Can you work these out from the model? Positions are in its coordinate system, mm. A direction names the side the tool comes from. Give positions to 0.01 mm unless a question says otherwise; leave off trailing zeros. Order: outer loops, then holes, each group sorted by start corner. A loop starts at its lowest first (then second) coordinate and runs counter-clockwise, first axis right, second up. Notation, with made-up numbers: (24.5, 62) - (29.5, 62) arc R12 cw to (29.5, 73) - close; hole circle Ø1 at (34.25, 3.25). An arc over 180 degrees is marked (long way). Use one line per item in the form item = value. Start each with the question number.
1) Which directions (+Z, -Z, +X, -X, +Y, -Y) give clear straight access to the entire face, cutting with the end or side of a thin tool? Please do faces 4 (the flat face through (1.2, -1.2, 5.85)), 5 (the flat face through (-1, -1, 6.35)).
2) Suppose I cut it at C-C, the plane z = 2.5. Write out the boundary of the cut face in (x, y), and give its area (3 significant figures).
3) We'd pull the mould along Y, two halves only. Please class faces 1 (the flat face through (-1, 1, 6.35)), 2 (the flat face through (0, 0, 6.1)), 3 (the cylindrical face through (2.65, 0.83, 6.1)): released by +Y, released by -Y, zero draft, split by the parting line, or undercut.
4) For pin 1 (1.5 mm diameter, centred on x = 1.5, z = 1, fed in from -Y); pin 2 (1.5 mm diameter, centred on y = 0, z = 4.5, fed in from +X); pin 3 (2 mm diameter, centred on x = -2, z = 4.5, fed in from -Y), each with a flat end and sliding along its axis, tell me the tip position at first contact or that it passes through.
5) Suppose I cut it at A-A, the plane x = 0. Write out the boundary of the cut face in (y, z) (3 decimals), and give its area (3 significant figures).
6) Please list where these lines run through material, in increasing order: probe 1 along Z at (x, y) = (-0.75, 2.5); probe 2 along Z at (x, y) = (-0.15, -0.5); probe 3 along X at (y, z) = (-0.35, 5.5).
7) Suppose I cut it at D-D, the plane y = 0.9. Write out the boundary of the cut face in (x, z) (3 decimals), and give its area (3 significant figures).
```python
from build123d import *

# Parameters (mm, degrees)
SKETCH1_R               = 1.5
BOSS_EXTRUDE1_DEPTH     = 6.35
SKETCH3_R               = 2.775
BOSS_EXTRUDE3_DEPTH     = 0.5
SKETCH4_W               = 0.5
SKETCH4_H               = 6.00854879
SKETCH4_W_2             = 6.00854879
SKETCH4_H_2             = 0.5
CUT_EXTRUDE_THIN1_DEPTH = 0.25


with BuildPart() as part:
    # Sketch1 → Boss-Extrude1 (new body)
    with BuildSketch(Plane.XY):
        Circle(SKETCH1_R)
    extrude(amount=BOSS_EXTRUDE1_DEPTH)

    # Sketch3 → Boss-Extrude3 (add)
    with BuildSketch(Plane.XY.offset(6.35)):
        Circle(SKETCH3_R)
    extrude(amount=-BOSS_EXTRUDE3_DEPTH)

    # Sketch4 → Cut-Extrude-Thin1 (cut)
    with BuildSketch(Plane.XY.offset(6.35)):
        Rectangle(SKETCH4_W, SKETCH4_H)
        Rectangle(SKETCH4_W_2, SKETCH4_H_2)
    extrude(amount=-CUT_EXTRUDE_THIN1_DEPTH, mode=Mode.SUBTRACT)


solid = part.part
```
Result sheet:
q1.face_4 = -Z
q1.face_5 = +Z, +X, -X, +Y, -Y
q2.outline = circle Ø3 at (0, 0)
q2.area = 7.07 mm²
q3.face_1 = zero draft
q3.face_2 = undercut
q3.face_3 = split by the parting line
q4.pin_1 = -1.3
q4.pin_2 = 1.5
q4.pin_3 = -1.12
q5.outline = (-2.775, 5.85) - (-1.5, 5.85) - (-1.5, 0) - (1.5, 0) - (1.5, 5.85) - (2.775, 5.85) - (2.775, 6.1) - (-2.775, 6.1) - close
q5.area = 18.9 mm²
q6.probe_1 = 5.85 to 6.35
q6.probe_2 = 0 to 6.1
q6.probe_3 = -1.46 to 1.46
q7.outline = (-2.625, 5.85) - (-1.2, 5.85) - (-1.2, 0) - (1.2, 0) - (1.2, 5.85) - (2.625, 5.85) - (2.625, 6.35) - (0.25, 6.35) - (0.25, 6.1) - (-0.25, 6.1) - (-0.25, 6.35) - (-2.625, 6.35) - close
q7.area = 16.5 mm²
